from build123d import *

# Parameters (mm, degrees)
SKETCH1_W                    = 43
SKETCH1_H                    = 50
BASE_FLANGE1_DEPTH           = 1
SKETCH2_R                    = 11.05
SKETCH2_R_2                  = 1.75
CUT_EXTRUDE1_DEPTH           = 50.749371855
EDGE_FLANGE1_STRIP_W         = 5.4732
EDGE_FLANGE1_STRIP_H         = 1
EDGE_FLANGE1_STRIP_CUT_DEPTH = 50
EDGE_FLANGE1_DEPTH           = 50
CUT_EXTRUDE2_REACH           = 61.54
SKETCH8_R                    = 2.1
CHAMFER1_SIZE                = 5


# Sheet-metal steps are written as plain solids
with BuildPart() as part:
    # Sketch1 → Base-Flange1 (new body)
    with BuildSketch(Plane(origin=(0, 0, 0), x_dir=(1, 0, 0), z_dir=(0, 1, 0))):
        with Locations((21.5, 0)):
            Rectangle(SKETCH1_W, SKETCH1_H)
    extrude(amount=-BASE_FLANGE1_DEPTH)

    # Sketch2 → Cut-Extrude1 (cut, through all)
    with BuildSketch(Plane(origin=(0, 0, 0), x_dir=(1, 0, 0), z_dir=(0, 1, 0))):
        with Locations(Location((21, 0, 0), (0, 0, 270))):
            Circle(SKETCH2_R)
        with Locations(Location((5.5, 15.5, 0), (0, 0, 270))):
            Circle(SKETCH2_R_2)
        with Locations(Location((36.5, 15.5, 0), (0, 0, 270))):
            Circle(SKETCH2_R_2)
        with Locations(Location((36.5, -15.5, 0), (0, 0, 270))):
            Circle(SKETCH2_R_2)
        with Locations(Location((5.5, -15.5, 0), (0, 0, 270))):
            Circle(SKETCH2_R_2)
    extrude(amount=-CUT_EXTRUDE1_DEPTH, mode=Mode.SUBTRACT)

    # Edge-Flange1 strip (across the edge) → Edge-Flange1 strip cut (cut)
    with BuildSketch(Plane(origin=(43, 0, 25), x_dir=(-1, 0, 0), z_dir=(0, 0, -1))):
        with Locations((-1, -0.5)):
            Rectangle(EDGE_FLANGE1_STRIP_W, EDGE_FLANGE1_STRIP_H)
    extrude(amount=EDGE_FLANGE1_STRIP_CUT_DEPTH, mode=Mode.SUBTRACT)

    # Edge-Flange1 section (across the edge) → Edge-Flange1 (add)
    with BuildSketch(Plane(origin=(43, 0, 25), x_dir=(-1, 0, 0), z_dir=(0, 0, -1))):
        with BuildLine():
            Line((0, 0.7366), (0, 34))
            Line((0, 34), (1, 34))
            Line((1, 34), (1, 0.7366))
            ThreePointArc((1, 0.7366), (1.215745145, 0.215745145), (1.7366, 0))
            Line((1.7366, 0), (1.7366, -1))
            ThreePointArc((1.7366, -1), (0.508638364, -0.491361636), (0, 0.7366))
        make_face()
    extrude(amount=EDGE_FLANGE1_DEPTH)

    # Sketch8 → Cut-Extrude2 (cut, up to next)
    with BuildSketch(Plane.ZY.offset(-42), mode=Mode.PRIVATE) as cut_extrude2_sk1:
        with Locations(Location((20, 29, 0), (0, 0, 270))):
            Circle(SKETCH8_R)
    cut_extrude2_tool1 = extrude(cut_extrude2_sk1.sketch, amount=-CUT_EXTRUDE2_REACH, mode=Mode.PRIVATE) & part.part
    # Sketch8 → Cut-Extrude2 (cut, up to next)
    with BuildSketch(Plane.ZY.offset(-42), mode=Mode.PRIVATE) as cut_extrude2_sk2:
        with Locations(Location((-20, 29, 0), (0, 0, 270))):
            Circle(SKETCH8_R)
    cut_extrude2_tool2 = extrude(cut_extrude2_sk2.sketch, amount=-CUT_EXTRUDE2_REACH, mode=Mode.PRIVATE) & part.part
    add(cut_extrude2_tool1.solids().sort_by_distance((42, 29, 20))[0], mode=Mode.SUBTRACT)
    add(cut_extrude2_tool2.solids().sort_by_distance((42, 29, -20))[0], mode=Mode.SUBTRACT)

    # Chamfer1
    chamfer1_edges = [part.edges().sort_by_distance(p)[0] for p in [
        (0, -0.5, -25),
        (0, -0.5, 25),
    ]]
    chamfer(chamfer1_edges, length=CHAMFER1_SIZE)


solid = part.part
Can you work these out from the model? Positions are in its coordinate system, mm. A direction names the side the tool comes from. Round coordinates to 2 decimals unless told otherwise and drop trailing zeros. Loops run counter-clockwise (first coordinate to the right, second up) from the corner with the lowest first, then second, coordinate; pieces in that order, holes last. Notation, with made-up numbers: (-22.75, -16) - (19.25, -16) arc R24 cw to (19.25, 17) - close; hole circle Ø3 at (57.5, 28). An arc over 180 degrees is marked (long way). Use CSV: the item, a comma, the result in double quotes. Start each with the question number.
1) If we section it at D-D on z = 3.5: Write out the boundary of the cut face in (x, y).
2) For faces 1 (the flat face through (42, 18, 0)), 2 (the cylindrical face through (3.95, -0.49, 16.31)), which set-ups out of +Z, -Z, +X, -X, +Y, -Y let a thin tool reach every point of the face, with its end or its side?
3) If we section it at A-A on x = 36.5: Write out the boundary of the cut face in (y, z), plus the area to 3 significant figures.
4) We'd pull the mould along Z, two halves only. Please class faces 3 (the flat face through (11, -1, -6)), 4 (the cylindrical face through (35.83, -0.493, 17.117)), 5 (the flat face through (2.5, -0.5, 22.5)): released by +Z, released by -Z, zero draft, split by the parting line, or undercut.
5) Please list where these lines run through material, in increasing order: probe 1 along X at (y, z) = (-0.7, -15.5); probe 2 along X at (y, z) = (7, 22.5); probe 3 along X at (y, z) = (-0.2, 15.5). Write a range as [from, to].
6) For pin 1 Ø5.5 at (y, z) = (29, -20) entering from -X; pin 2 Ø12.5 at (x, z) = (24, 6.5) entering from +Y; pin 3 Ø5.5 at (x, z) = (5.5, 15.5) entering from -Y; pin 4 Ø3 at (x, z) = (5.5, -15.5) entering from -Y, each with a flat end and sliding along its axis, tell me the tip position at first contact or that it passes through.
7) If we section it at B-B on z = 15.5: Write out the boundary of the cut face in (x, y), plus the area to 3 significant figures.
8) If we section it at C-C on x = 21: Write out the boundary of the cut face in (y, z), plus the area to 3 significant figures.
Geometry results:
1,outline,"(0, -1) - (10.52, -1) - (10.52, 0) - (0, 0) - close; (31.48, -1) - (41.26, -1) arc R1.74 ccw to (43, 0.74) - (43, 34) - (42, 34) - (42, 0.74) arc R0.74 cw to (41.26, 0) - (31.48, 0) - close"
2,face 1,"+Z, -Z, -X, +Y"
2,face 2,"+Y, -Y"
3,outline,"(-1, -25) - (0, -25) - (0, -17.25) - (-1, -17.25) - close; (-1, -13.75) - (0, -13.75) - (0, 13.75) - (-1, 13.75) - close; (-1, 17.25) - (0, 17.25) - (0, 25) - (-1, 25) - close"
3,area,"43.0 mm2"
4,face 3,"zero draft"
4,face 4,"undercut"
4,face 5,"released by +Z"
5,probe 1,"x = [0, 3.75], [7.25, 34.75], [38.25, 42.24]"
5,probe 2,"x = [42, 43]"
5,probe 3,"x = [0, 3.75], [7.25, 34.75], [38.25, 42.73]"
6,pin 1,"stops at x = 42"
6,pin 2,"stops at y = 0"
6,pin 3,"stops at y = -1"
6,pin 4,"passes through"
7,outline,"(0, -1) - (3.75, -1) - (3.75, 0) - (0, 0) - close; (7.25, -1) - (34.75, -1) - (34.75, 0) - (7.25, 0) - close; (38.25, -1) - (41.26, -1) arc R1.74 ccw to (43, 0.74) - (43, 34) - (42, 34) - (42, 0.74) arc R0.74 cw to (41.26, 0) - (38.25, 0) - close"
7,area,"69.5 mm2"
8,outline,"(-1, -25) - (0, -25) - (0, -11.05) - (-1, -11.05) - close; (-1, 11.05) - (0, 11.05) - (0, 25) - (-1, 25) - close"
8,area,"27.9 mm2"
